Check sheet for the modelled part. Datum: model origin and axes. Units: mm. A direction names the side the tool comes from. Give positions to 0.01 mm unless a question says otherwise; leave off trailing zeros. Order: outer loops, then holes, each group sorted by start corner. A loop starts at its lowest first (then second) coordinate and runs counter-clockwise, first axis right, second up. Notation, with made-up numbers: (-34, -16) -> (14, -16) arc R14 ccw to (14, -3) -> close; hole circle Ø1 at (85, -28.5). An arc over 180 degrees is marked (long way). Write each question's results on one line, items separated by ' | '.
from build123d import *

# Parameters (mm, degrees)
F0_W      = 16
F0_H      = 8
F1_DEPTH  = 11
F3_DEPTH  = 11
F5_DEPTH  = 8
F6_W      = 10
F6_H      = 7
F7_DEPTH  = 25.4
F9_DEPTH  = 25.4
F10_R     = 2.9921817394
F11_DEPTH = 25.4
F12_R     = 1.0573915373
F13_DEPTH = 25.4


with BuildPart() as f1:
    # F0 (on Top) → F1 (new body)
    with BuildSketch(Plane.XY):
        with Locations((8, 4)):
            Rectangle(F0_W, F0_H)
    extrude(amount=F1_DEPTH)

    # F2 (on face) → F3 (join)
    with BuildSketch(Plane.XY.offset(11)):
        with BuildLine():
            Line((16, 7), (16, 1))
            ThreePointArc((16, 1), (18.1213203436, 1.8786796564), (19, 4))
            ThreePointArc((19, 4), (18.1213203436, 6.1213203436), (16, 7))
        make_face()
    extrude(amount=-F3_DEPTH)

    # F4 (on face) → F5 (join)
    with BuildSketch(Plane(origin=(0, 8, 0), x_dir=(-1, 0, 0), z_dir=(0, 1, 0))):
        with BuildLine():
            Line((-16, 11), (0, 11))
            ThreePointArc((0, 11), (-8, 12.9014484288), (-16, 11))
        make_face()
    extrude(amount=-F5_DEPTH)

    # F6 (on face) → F7 (cut)
    with BuildSketch(Plane(origin=(0, 8, 0), x_dir=(-1, 0, 0), z_dir=(0, 1, 0))):
        with Locations((-8, 3.5)):
            Rectangle(F6_W, F6_H)
    extrude(amount=-F7_DEPTH, mode=Mode.SUBTRACT)

    # F8 (on face) → F9 (cut)
    with BuildSketch(Plane(origin=(0, 8, 0), x_dir=(-1, 0, 0), z_dir=(0, 1, 0))):
        with BuildLine():
            Line((-13, 7), (-3, 7))
            ThreePointArc((-3, 7), (-8, 11.2036427481), (-13, 7))
        make_face()
    extrude(amount=-F9_DEPTH, mode=Mode.SUBTRACT)

    # F10 (on face) → F11 (cut)
    with BuildSketch(Plane.XY.offset(11)):
        with Locations((16, 4)):
            Circle(F10_R)
    extrude(amount=F11_DEPTH, mode=Mode.SUBTRACT)

    # F12 (on face) → F13 (cut)
    with BuildSketch(Plane.XY.offset(11)):
        with Locations((16, 4)):
            Circle(F12_R)
    extrude(amount=-F13_DEPTH, mode=Mode.SUBTRACT)


solid = f1.part
1. Section check A-A on z = 5.5. Record the cut outline in (x, y).
Verdict:
outline: (0, 0) -> (3, 0) -> (3, 8) -> (0, 8) -> close; (13, 0) -> (16, 0) -> (16, 1) arc R3 ccw to (16, 7) -> (16, 8) -> (13, 8) -> close; hole circle Ø2.11 at (16, 4)
2. Material ranges on probe 1 along X at (y, z) = (7.25, 2.5); probe 2 along X at (y, z) = (4.5, 4.25); probe 3 along X at (y, z) = (4.25, 1), recorded low to high. Write a range as from..to.
Verdict:
probe 1: x = 0..3, 13..16 | probe 2: x = 0..3, 13..15.07, 16.93..18.96 | probe 3: x = 0..3, 13..14.97, 17.03..18.99
3. Mould release check, pull along Y, two halves, no side actions. Record for faces 1 (the flat face through (10, 0, 11)), 2 (the flat face through (0, 4, 5)), 3 (the cylindrical face through (14.944, 4.046, 5.577)): +Y half, -Y half, draft (parallel to the pull), parting line (faces both ways), or undercut.
Verdict:
face 1: -Y half | face 2: draft | face 3: undercut
4. Section check D-D on z = 8. Record the cut outline in (x, y), then the cut area to 3 significant figures.
Verdict:
outline: (0, 0) -> (3.28, 0) -> (3.28, 8) -> (0, 8) -> close; (12.72, 0) -> (16, 0) -> (16, 1) arc R3 ccw to (16, 7) -> (16, 8) -> (12.72, 8) -> close; hole circle Ø2.11 at (16, 4) | area: 63.1 mm^2
5. Section check C-C on y = 5.5. Record the cut outline in (x, z).
Verdict:
outline: (0, 0) -> (3, 0) -> (3, 7) arc R5.08 cw to (13, 7) -> (13, 0) -> (18.6, 0) -> (18.6, 11) -> (13.41, 11) -> (13.41, 12.06) arc R17.78 ccw to (0, 11) -> close
6. Access from +Z, -Z, +X, -X, +Y, -Y to the whole of each face (thin tool, end or side, straight path). Record for faces 4 (the flat face through (3, 4, 3)), 5 (the flat face through (16, 7.5, 5.4)), 6 (the flat face through (16, 0.5, 5.4)), 7 (the cylindrical face through (13.01, 4.07, 11.45)).
Verdict:
face 4: -Z, +Y, -Y | face 5: +Z, -Z, +X, +Y | face 6: +Z, -Z, +X, -Y | face 7: +Z, +X
7. Gauge pin test, flat end, axial feed: pin 1 Ø0.8 at (y, z) = (0.5, 6.5) entering from +X. Record the tip position at first contact, or that the pin passes through.
Verdict:
pin 1: stops at x = 16
8. Section check B-B on x = 16.5. Record the cut outline in (y, z), then the cut area to 3 significant figures.
Verdict:
outline: (1.04, 0) -> (3.07, 0) -> (3.07, 11) -> (1.04, 11) -> close; (4.93, 0) -> (6.96, 0) -> (6.96, 11) -> (4.93, 11) -> close | area: 44.6 mm^2
